from build123d import *

# Parameters (mm, degrees)
SKETCH_1_W          = 36
SKETCH_1_H          = 120
EXTRUDE_1_DEPTH     = 20
SKETCH_2_W          = 30
SKETCH_2_H          = 76.64229125
CUT_EXTRUDE_1_DEPTH = 20
SKETCH_3_W          = 53.751349406
SKETCH_3_H          = 17.737070837
SKETCH_3_W_2        = 54.426052537
SKETCH_3_H_2        = 11.321534577
CUT_EXTRUDE_2_DEPTH = 30
SKETCH_5_R          = 2
CUT_EXTRUDE_3_DEPTH = 70


with BuildPart() as part:
    # 草图1 → 凸台-拉伸1 (new body)
    with BuildSketch(Plane(origin=(0, 0, 0), x_dir=(1, 0, 0), z_dir=(0, 1, 0))):
        Rectangle(SKETCH_1_W, SKETCH_1_H)
    extrude(amount=EXTRUDE_1_DEPTH)

    # 草图2 → 切除-拉伸1 (cut)
    with BuildSketch(Plane(origin=(0, 20, 0), x_dir=(1, 0, 0), z_dir=(0, 1, 0))):
        with Locations((0, -38.321145625)):
            Rectangle(SKETCH_2_W, SKETCH_2_H)
    extrude(amount=-CUT_EXTRUDE_1_DEPTH, mode=Mode.SUBTRACT)

    # 草图3 → 切除-拉伸2 (cut)
    with BuildSketch(Plane(origin=(0, 0, -60), x_dir=(-1, 0, 0), z_dir=(0, 0, -1))):
        with Locations((-0.187417536, -3.868535419)):
            Rectangle(SKETCH_3_W, SKETCH_3_H)
        with Locations((0.074967015, 20.660767289)):
            Rectangle(SKETCH_3_W_2, SKETCH_3_H_2)
    extrude(amount=-CUT_EXTRUDE_2_DEPTH, mode=Mode.SUBTRACT)

    # 草图5 → 切除-拉伸3 (cut)
    with BuildSketch(Plane(origin=(18, 0, 0), x_dir=(0, 0, -1), z_dir=(1, 0, 0))):
        with Locations((-50, 10)):
            Circle(SKETCH_5_R)
    extrude(amount=-CUT_EXTRUDE_3_DEPTH, mode=Mode.SUBTRACT)


solid = part.part
Design review of the part built by this model. Coordinates are the model's own, in mm. A direction names the side the tool comes from. Coordinates: 2 decimals unless noted, no trailing zeros. Loops run counter-clockwise (first coordinate to the right, second up) from the corner with the lowest first, then second, coordinate; pieces in that order, holes last. Notation, with made-up numbers: (-13.5, 51) -> (18.5, 51) arc R17 cw to (18.5, 83) -> close; hole circle Ø1 at (-35, -5.75). An arc over 180 degrees is marked (long way). Use a Markdown table: item, result. Add a question column.
Item 1: Wall thickness on L1, parallel to X at y = 4.5, z = 45; L2, parallel to Y at x = 15.6, z = 50; L3, parallel to Z at x = 3, y = 4.75: over which ranges is each line inside the solid? List them lowest first. Write a range as from..to.
Item 2: The part is to be moulded in two halves that separate along X. For faces 1 (the flat face through (0, 10, 0)), 2 (the flat face through (-15, 10, 30)), 3 (the flat face through (18, 10, 1)), 4 (the flat face through (0, 10, -60)), say which applies: +X half, -X half, draft (parallel to the pull), parting line (faces both ways), or undercut.
Item 3: We need section B-B, the plane z = 37. Write out the cut boundary in (x, y), and give its area (3 significant figures).
Item 4: Clearance check with flat-ended pins moving along their axes: P1, Ø1, axis at x = 13, y = 11.5, coming from the +Z side; P2, Ø9, axis at x = -1, z = -40.5, coming from the +Y side; P3, Ø2.5, axis at x = -5, y = 2.5, coming from the -Z side. State where each tip first meets the part, or that it passes through.
Item 5: We need section D-D, the plane x = 12.5. Write out the cut boundary in (y, z).
Item 6: We need section C-C, the plane z = 50. Write out the cut boundary in (x, y).
Item 7: Machinability: for faces 5 (the flat face through (15, 10, 30)), 6 (the flat face through (0, 5, -45)), 7 (the cylindrical face through (-16.479, 11.352, 51.474)), 8 (the flat face through (0, 15, -45)), 9 (the flat face through (-17, 10, 60)), which of the approach directions +Z, -Z, +X, -X, +Y, -Y give a long, thin tool a straight path to every point of the face, cutting with its end or side? Answer none if there is none.
Item 8: We need section A-A, the plane y = 10. Write out the cut boundary in (x, z).
Numbers:
| question | item | result |
|---|---|---|
| 1 | L1 | x = -18..-15, 15..18 |
| 1 | L2 | y = 0..8, 12..20 |
| 1 | L3 | z = -30..0 |
| 2 | face 1 | undercut |
| 2 | face 2 | undercut |
| 2 | face 3 | +X half |
| 2 | face 4 | draft |
| 3 | outline | (-18, 0) -> (-15, 0) -> (-15, 20) -> (-18, 20) -> close; (15, 0) -> (18, 0) -> (18, 20) -> (15, 20) -> close |
| 3 | area | 120 mm^2 |
| 4 | P1 | stops at z = 0 |
| 4 | P2 | stops at y = 15 |
| 4 | P3 | stops at z = -30 |
| 5 | outline | (0, -30) -> (5, -30) -> (5, -60) -> (15, -60) -> (15, -30) -> (20, -30) -> (20, 0) -> (0, 0) -> close |
| 6 | outline | (-18, 0) -> (-15, 0) -> (-15, 8) -> (-18, 8) -> close; (-18, 12) -> (-15, 12) -> (-15, 20) -> (-18, 20) -> close; (15, 0) -> (18, 0) -> (18, 8) -> (15, 8) -> close; (15, 12) -> (18, 12) -> (18, 20) -> (15, 20) -> close |
| 7 | face 5 | +Z, +Y, -Y |
| 7 | face 6 | -Z, +X, -X, -Y |
| 7 | face 7 | +X, -X |
| 7 | face 8 | -Z, +X, -X, +Y |
| 7 | face 9 | +Z, +X, -X, +Y, -Y |
| 8 | outline | (-18, -60) -> (18, -60) -> (18, 48) -> (15, 48) -> (15, 0) -> (-15, 0) -> (-15, 48) -> (-18, 48) -> close; (-18, 52) -> (-15, 52) -> (-15, 60) -> (-18, 60) -> close; (15, 52) -> (18, 52) -> (18, 60) -> (15, 60) -> close |
